Verification items for the finished model (mm, model axes). Face numbers are marked on the shaded views. A direction names the side the tool comes from. Coordinates: 2 decimals unless noted, no trailing zeros. Loops run counter-clockwise (first coordinate to the right, second up) from the corner with the lowest first, then second, coordinate; pieces in that order, holes last. Notation, with made-up numbers: (64.25, 73.25) -> (77.25, 73.25) arc R28 cw to (77.25, 97.25) -> close; hole circle Ø3 at (53.25, 29.5). An arc over 180 degrees is marked (long way). Use CSV: the item, a comma, the result in double quotes. Start each with the question number.
```python
from build123d import *

# Parameters (mm, degrees)
BOSS_EXTRUDE1_DEPTH = 6.35
SKETCH3_R           = 1.5
SKETCH3_R_2         = 7
CUT_EXTRUDE1_DEPTH  = 7.35
FILLET1_R           = 20


with BuildPart() as part:
    # Sketch2 → Boss-Extrude1 (new body)
    with BuildSketch(Plane(origin=(0, 0, 0), x_dir=(1, 0, 0), z_dir=(0, 1, 0))):
        Polygon((0, 0), (44.15, 0), (44.15, -5.842), (63.15, -5.842), (63.15, 0), (68.15, 0), (68.15, 10), (10, 74.5), (0, 74.5), (0, 69.5), (-5.87, 69.5), (-5.87, 50.5), (0, 50.5), align=None)
    extrude(amount=BOSS_EXTRUDE1_DEPTH)

    # Sketch3 → Cut-Extrude1 (cut, through all)
    with BuildSketch(Plane(origin=(0, 6.35, 0), x_dir=(1, 0, 0), z_dir=(0, 1, 0))):
        with Locations((0, 69.5)):
            Circle(SKETCH3_R)
        with Locations((0, 50.5)):
            Circle(SKETCH3_R)
        with Locations((44.15, 0)):
            Circle(SKETCH3_R)
        with Locations((63.15, 0)):
            Circle(SKETCH3_R)
        with Locations((0, 20)):
            Circle(SKETCH3_R_2)
        with Locations((13.65, 0)):
            Circle(SKETCH3_R_2)
    extrude(amount=-CUT_EXTRUDE1_DEPTH, mode=Mode.SUBTRACT)

    # Fillet1
    fillet1_edges = [part.edges().sort_by_distance(p)[0] for p in [
        (10, 3.175, -74.5),
        (68.15, 3.175, -10),
    ]]
    fillet(fillet1_edges, radius=FILLET1_R)


solid = part.part
```
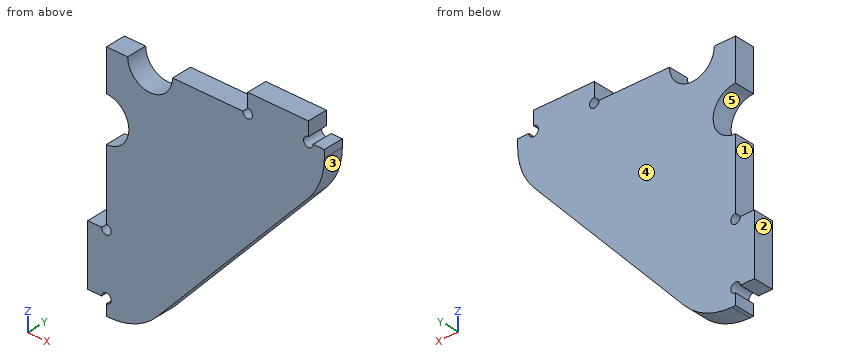
1. Cross-section at B-B, the plane y = 1. Record the boundary of the cut face in (x, z).
2. Set-up check for the marked faces 1 and 2: record each of +Z, -Z, +X, -X, +Y, -Y from which the full face is reachable in a straight line by a thin tool's end or side.
3. Cross-section at D-D, the plane x = 25.5. Record the boundary of the cut face in (y, z).
4. Cross-section at A-A, the plane x = 3. Record the boundary of the cut face in (y, z).
5. Depth check by flat-ended pin: pin 1 (3 mm diameter, centred on y = 1.5, z = -73.5, fed in from -X); pin 2 (1 mm diameter, centred on x = 35, y = 4.5, fed in from -Z); pin 3 (1.9 mm diameter, centred on x = 27.5, y = 4, fed in from +Z); pin 4 (1.8 mm diameter, centred on x = 0, z = -50.5, fed in from -Y). Enter the tip coordinate at first touch or a pass-through.
6. Cross-section at C-C, the plane z = -47. Record the boundary of the cut face in (x, y).
7. Release check for a two-part mould opening along Z. For the marked faces 3, 4 and 5 record: released by +Z, released by -Z, zero draft, split by the parting line, or undercut.
8. Scan lines: line 1 (X direction, y = 0.5, z = -2.5); line 2 (X direction, y = 0.75, z = 3); line 3 (X direction, y = 1.75, z = -6). Record each from-to range of solid material in increasing order.
Solution:
1,outline,"(-5.87, -69.5) -> (-1.5, -69.5) arc R1.5 cw (long way) to (0, -71) -> (0, -74.5) -> (1.1, -74.5) arc R20 ccw to (15.96, -67.89) -> (63, -15.71) arc R20 ccw to (68.15, -2.32) -> (68.15, 0) -> (64.65, 0) arc R1.5 cw (long way) to (63.15, 1.5) -> (63.15, 5.84) -> (44.15, 5.84) -> (44.15, 1.5) arc R1.5 cw (long way) to (42.65, 0) -> (20.65, 0) arc R7 cw to (6.65, 0) -> (0, 0) -> (0, -13) arc R7 cw to (0, -27) -> (0, -49) arc R1.5 cw (long way) to (-1.5, -50.5) -> (-5.87, -50.5) -> close"
2,face 1,"+Z, -X, +Y, -Y"
2,face 2,"+Z, -Z, -X, +Y, -Y"
3,outline,"(0, -57.31) -> (6.35, -57.31) -> (6.35, 0) -> (0, 0) -> close"
4,outline,"(0, -74.41) -> (6.35, -74.41) -> (6.35, -26.32) -> (0, -26.32) -> close; (0, -13.68) -> (6.35, -13.68) -> (6.35, 0) -> (0, 0) -> close"
5,pin 1,"stops at x = 0"
5,pin 2,"stops at z = -47.32"
5,pin 3,"stops at z = 0"
5,pin 4,"passes through"
6,outline,"(0, 0) -> (34.79, 0) -> (34.79, 6.35) -> (0, 6.35) -> close"
7,face 3,"released by -Z"
7,face 4,"zero draft"
7,face 5,"undercut"
8,line 1,"x = 0 to 7.11, 20.19 to 68.15"
8,line 2,"x = 44.15 to 63.15"
8,line 3,"x = 0 to 10.04, 17.26 to 67.81"
